Design review of the part built by this model. Coordinates are the model's own, in mm. Round coordinates to 2 decimals unless told otherwise and drop trailing zeros. Loops run counter-clockwise (first coordinate to the right, second up) from the corner with the lowest first, then second, coordinate; pieces in that order, holes last. Notation, with made-up numbers: (29.25, -13.75) - (60.25, -13.75) arc R26 cw to (60.25, 25.25) - close; hole circle Ø9 at (-11, 4). An arc over 180 degrees is marked (long way). Use one line per item in the form item = value. Start each with the question number.
(1) We need section B-B, the plane z = 3.5. Write out the cut boundary in (x, y), then the cut area to 3 significant figures.
(2) We need section D-D, the plane z = 18.5. Write out the cut boundary in (x, y), then the cut area to 3 significant figures.
(3) Wall thickness on probe 1 along Z at (x, y) = (-9, -0.25); probe 2 along X at (y, z) = (-6, 3); probe 3 along Z at (x, y) = (-3.5, -2.5): over which ranges is each line inside the solid? List them lowest first. Write a range as [from, to].
(4) For pin 1 (4 mm diameter, centred on y = -1, z = -12, fed in from -X); pin 2 (4 mm diameter, centred on x = 9.5, y = -4, fed in from -Z); pin 3 (2 mm diameter, centred on x = 12, y = -5.5, fed in from +Z), all flat-tipped, find the tip position at first contact; note any pin that passes through.
(5) We need section C-C, the plane x = -7.5. Write out the cut boundary in (y, z), then the cut area to 3 significant figures.
(6) We need section A-A, the plane y = -4.75. Write out the cut boundary in (x, z), then the cut area to 3 significant figures.
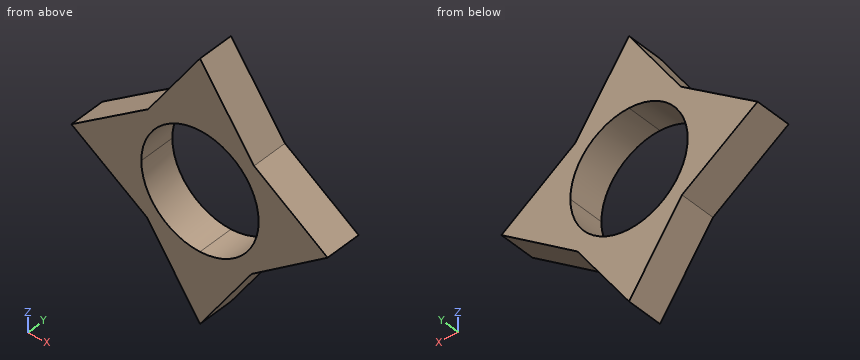
from build123d import *

# Parameters (mm, degrees)
F1_DEPTH = 6.9342


with BuildPart() as f1:
    # F0 (on Front) → F1 (new body)
    with BuildSketch(Plane.XZ):
        with BuildLine():
            ThreePointArc((-11.0998, 0), (-7.848744, 7.848744), (0, 11.0998))
            Line((0, 11.0998), (0, 24.298547))
            Line((0, 24.298547), (-9.813829, 10.06805))
            Line((-9.813829, 10.06805), (-24.327461, 0))
            Line((-24.327461, 0), (-11.0998, 0))
        make_face()
        with BuildLine():
            Line((0, 24.298547), (0, 11.0998))
            ThreePointArc((0, 11.0998), (7.848744, 7.848744), (11.0998, 0))
            Line((11.0998, 0), (24.14246, 0))
            Line((24.14246, 0), (10.217335, 9.78862))
            Line((10.217335, 9.78862), (0, 24.298547))
        make_face()
        with BuildLine():
            ThreePointArc((0, -11.0998), (-7.848744, -7.848744), (-11.0998, 0))
            Line((-11.0998, 0), (-24.327461, 0))
            Line((-24.327461, 0), (-10.020223, -9.861334))
            Line((-10.020223, -9.861334), (0, -24.327463))
            Line((0, -24.327463), (0, -11.0998))
        make_face()
        with BuildLine():
            Line((24.14246, 0), (11.0998, 0))
            ThreePointArc((11.0998, 0), (7.848744, -7.848744), (0, -11.0998))
            Line((0, -11.0998), (0, -24.327463))
            Line((0, -24.327463), (9.758095, -10.243655))
            Line((9.758095, -10.243655), (24.14246, 0))
        make_face()
    extrude(amount=F1_DEPTH)


solid = f1.part
Data:
q1.outline = (-19.28, -6.93) - (-10.53, -6.93) - (-10.53, 0) - (-19.28, 0) - close; (10.53, -6.93) - (19.16, -6.93) - (19.16, 0) - (10.53, 0) - close
q1.area = 121 mm^2
q2.outline = (-4, -6.93) - (4.08, -6.93) - (4.08, 0) - (-4, 0) - close
q2.area = 56.0 mm^2
q3.probe_1 = [-11.33, -6.5], [6.5, 11.25]
q3.probe_2 = [-20, -10.69], [10.69, 19.87]
q3.probe_3 = [-19.27, -10.53], [10.53, 19.22]
q4.pin_1 = -9.92
q4.pin_2 = -13.5
q4.pin_3 = 9.24
q5.outline = (-6.93, -13.5) - (0, -13.5) - (0, -8.18) - (-6.93, -8.18) - close; (-6.93, 8.18) - (0, 8.18) - (0, 13.42) - (-6.93, 13.42) - close
q5.area = 73.2 mm^2
q6.outline = (-24.33, 0) - (-10.02, -9.86) - (0, -24.33) - (9.76, -10.24) - (24.14, 0) - (10.22, 9.79) - (0, 24.3) - (-9.81, 10.07) - close; hole (-11.1, 0) arc R11.1 ccw to (0, -11.1) arc R11.1 ccw to (11.1, 0) arc R11.1 ccw to (0, 11.1) arc R11.1 ccw to start
q6.area = 581 mm^2
